Verification items for the finished model (mm, model axes). Round coordinates to 2 decimals unless told otherwise and drop trailing zeros. Order: outer loops, then holes, each group sorted by start corner. A loop starts at its lowest first (then second) coordinate and runs counter-clockwise, first axis right, second up. Notation, with made-up numbers: (10, -6.75) -> (41, -6.75) arc R20 ccw to (41, 9.25) -> close; hole circle Ø9 at (35, -36). An arc over 180 degrees is marked (long way). Put each result on its own line as item: value.
from build123d import *

# Parameters (mm, degrees)
F1_DEPTH = 6.35


with BuildPart() as f1:
    # F0 (on Top) → F1 (new body)
    with BuildSketch(Plane.XY):
        with BuildLine():
            ThreePointArc((-18.7706, 3.2507038684), (-1.6313445375, -18.98002147), (19.05, 0))
            ThreePointArc((19.05, 0), (18.98002147, 1.6313445375), (18.7706, 3.2507038684))
            Line((18.7706, 3.2507038684), (9.222893546, 3.2507038684))
            ThreePointArc((9.222893546, 3.2507038684), (9.6389708213, 1.6489640709), (9.779, 0))
            ThreePointArc((9.779, 0), (-1.6489640709, -9.6389708213), (-9.222893546, 3.2507038684))
            Line((-9.222893546, 3.2507038684), (-18.7706, 3.2507038684))
        make_face()
        with BuildLine():
            Line((-9.3853, 57.1878519342), (-18.7706, 3.2507038684))
            ThreePointArc((-18.7706, 3.2507038684), (-12.2673671036, 14.5744366734), (0, 19.05))
            Line((0, 19.05), (0, 46.0375))
            ThreePointArc((0, 46.0375), (-7.2872183367, 49.4288164482), (-9.3853, 57.1878519342))
        make_face()
        with BuildLine():
            Line((9.222893546, 3.2507038684), (18.7706, 3.2507038684))
            ThreePointArc((18.7706, 3.2507038684), (12.2673671036, 14.5744366734), (0, 19.05))
            Line((0, 19.05), (0, 9.779))
            ThreePointArc((0, 9.779), (5.6497879549, 7.9817753078), (9.222893546, 3.2507038684))
        make_face()
        with BuildLine():
            ThreePointArc((0, 19.05), (12.2673671036, 14.5744366734), (18.7706, 3.2507038684))
            Line((18.7706, 3.2507038684), (9.3853, 57.1878519342))
            ThreePointArc((9.3853, 57.1878519342), (9.490010735, 56.3781722687), (9.525, 55.5625))
            ThreePointArc((9.525, 55.5625), (6.7351920908, 48.8273079092), (0, 46.0375))
            Line((0, 46.0375), (0, 19.05))
        make_face()
        with BuildLine():
            ThreePointArc((0, 19.05), (-12.2673671036, 14.5744366734), (-18.7706, 3.2507038684))
            Line((-18.7706, 3.2507038684), (-9.222893546, 3.2507038684))
            ThreePointArc((-9.222893546, 3.2507038684), (-5.6497879549, 7.9817753078), (0, 9.779))
            Line((0, 9.779), (0, 19.05))
        make_face()
        with BuildLine():
            Line((2.7274266425, 57.1878519342), (9.3853, 57.1878519342))
            ThreePointArc((9.3853, 57.1878519342), (0, 65.0875), (-9.3853, 57.1878519342))
            Line((-9.3853, 57.1878519342), (-2.7274266425, 57.1878519342))
            ThreePointArc((-2.7274266425, 57.1878519342), (0, 58.7375), (2.7274266425, 57.1878519342))
        make_face()
        with BuildLine():
            ThreePointArc((9.525, 55.5625), (9.490010735, 56.3781722687), (9.3853, 57.1878519342))
            Line((9.3853, 57.1878519342), (2.7274266425, 57.1878519342))
            ThreePointArc((2.7274266425, 57.1878519342), (3.0610622821, 56.4054250887), (3.175, 55.5625))
            ThreePointArc((3.175, 55.5625), (2.2450640303, 53.3174359697), (0, 52.3875))
            Line((0, 52.3875), (0, 46.0375))
            ThreePointArc((0, 46.0375), (6.7351920908, 48.8273079092), (9.525, 55.5625))
        make_face()
        with BuildLine():
            Line((-2.7274266425, 57.1878519342), (-9.3853, 57.1878519342))
            ThreePointArc((-9.3853, 57.1878519342), (-7.2872183367, 49.4288164482), (0, 46.0375))
            Line((0, 46.0375), (0, 52.3875))
            ThreePointArc((0, 52.3875), (-2.7605359435, 53.9940401489), (-2.7274266425, 57.1878519342))
        make_face()
    extrude(amount=F1_DEPTH)


solid = f1.part
Item 1: Section check B-B on x = -4. Record the boundary of the cut face in (y, z), then the cut area to 3 significant figures.
Check sheet entries:
outline: (-18.63, 0) -> (-8.92, 0) -> (-8.92, 6.35) -> (-18.63, 6.35) -> close; (8.92, 0) -> (64.21, 0) -> (64.21, 6.35) -> (8.92, 6.35) -> close
area: 413 mm^2
Item 2: Material ranges on L1, parallel to Y at x = 0, z = 2; L2, parallel to Y at x = 1.5, z = 0.5; L3, parallel to X at y = 22.5, z = 2, recorded low to high. Write a range as [from, to].
Check sheet entries:
L1: y = [-19.05, -9.78], [9.78, 52.39], [58.74, 65.09]
L2: y = [-18.99, -9.66], [9.66, 52.76], [58.36, 64.97]
L3: x = [-15.42, 15.42]
Item 3: Section check A-A on z = 5.25. State how many separate pieces and enclosed holes the cut face has, then the cut area to 3 significant figures.
Check sheet entries:
separate pieces: 1
enclosed holes: 2
area: 1,990 mm^2
Item 4: Section check C-C on y = 2. Record the boundary of the cut face in (x, z).
Check sheet entries:
outline: (-18.94, 0) -> (-9.57, 0) -> (-9.57, 6.35) -> (-18.94, 6.35) -> close; (9.57, 0) -> (18.94, 0) -> (18.94, 6.35) -> (9.57, 6.35) -> close
Item 5: Gauge pin test, flat ends, axial feed: pin 1 Ø2 at (y, z) = (10, 2.5) entering from +X; pin 2 Ø1 at (x, z) = (-3.5, 5.5) entering from -Y; pin 3 Ø2 at (x, z) = (-14.5, 4.5) entering from -Y. Record the tip position at first contact, or that the pin passes through.
Check sheet entries:
pin 1: stops at x = 17.77
pin 2: stops at y = -18.81
pin 3: stops at y = -13.44
Item 6: Section check D-D on y = 39.5. Record the boundary of the cut face in (x, z), then the cut area to 3 significant figures.
Check sheet entries:
outline: (-12.46, 0) -> (12.46, 0) -> (12.46, 6.35) -> (-12.46, 6.35) -> close
area: 158 mm^2
